```python
from build123d import *

# Parameters (mm, degrees)
SKETCH1_W           = 30
SKETCH1_H           = 239.95
BOSS_EXTRUDE1_DEPTH = 3.75
SKETCH2_W           = 30
SKETCH2_H           = 5
BOSS_EXTRUDE2_DEPTH = 20
SKETCH3_W           = 30
SKETCH3_H           = 5
BOSS_EXTRUDE3_DEPTH = 20
FILLET1_R           = 10
FILLET2_R           = 10


with BuildPart() as part:
    # Sketch1 → Boss-Extrude1 (new body, symmetric)
    with BuildSketch(Plane.XY):
        with Locations((0, 119.975)):
            Rectangle(SKETCH1_W, SKETCH1_H)
    extrude(amount=BOSS_EXTRUDE1_DEPTH, both=True)

    # Sketch2 → Boss-Extrude2 (add, symmetric)
    with BuildSketch(Plane.XY):
        with Locations((0, 2.5)):
            Rectangle(SKETCH2_W, SKETCH2_H)
    extrude(amount=BOSS_EXTRUDE2_DEPTH, both=True)

    # Sketch3 → Boss-Extrude3 (add, symmetric)
    with BuildSketch(Plane.XY):
        with Locations((0, 237.45)):
            Rectangle(SKETCH3_W, SKETCH3_H)
    extrude(amount=BOSS_EXTRUDE3_DEPTH, both=True)

    # Fillet1
    fillet1_edges = [part.edges().sort_by_distance(p)[0] for p in [
        (0, 234.95, 3.75),
        (0, 234.95, -3.75),
    ]]
    fillet(fillet1_edges, radius=FILLET1_R)

    # Fillet2
    fillet2_edges = [part.edges().sort_by_distance(p)[0] for p in [
        (0, 5, -3.75),
        (0, 5, 3.75),
    ]]
    fillet(fillet2_edges, radius=FILLET2_R)


solid = part.part
```
CAD build for the part. Positions are in the model's coordinates, mm. A direction names the side the tool comes from. Give positions to 0.01 mm unless a question says otherwise; leave off trailing zeros. Loops run counter-clockwise (first coordinate to the right, second up) from the corner with the lowest first, then second, coordinate; pieces in that order, holes last. Notation, with made-up numbers: (-27, 19.5) - (32, 19.5) arc R19 cw to (32, 31.5) - close; hole circle Ø9 at (27, 71). An arc over 180 degrees is marked (long way). Put each result on its own line as item: value.
Q1. Slice it at C-C (y = 46.5). Give the cut face in (x, z), plus the area to 3 significant figures.
Filled in:
outline: (-15, -3.75) - (15, -3.75) - (15, 3.75) - (-15, 3.75) - close
area: 225 mm²
Q2. Mould opens along X. For faces 4 (the face through (15, 111, 0)), 5 (the face through (0, 5, 17)), 6 (the face through (-15, 111, 0)) say: pulls with the +X half, pulls with the -X half, needs draft (parallel to the pull), parting line crosses it, or undercut.
Filled in:
face 4: pulls with the +X half
face 5: needs draft
face 6: pulls with the -X half
Q3. Probe line 1 along Y through (x, z) = (-8.25, 15); line 2 along Z through (x, y) = (8.25, 180); line 3 along Y through (x, z) = (-5.5, -11). List the from-to ranges inside material, lowest first.
Filled in:
line 1: y = 0 to 5, 234.95 to 239.95
line 2: z = -3.75 to 3.75
line 3: y = 0 to 5.39, 234.56 to 239.95
Q4. Slice it at B-B (z = -17). Give the cut face in (x, y).
Filled in:
outline: (-15, 0) - (15, 0) - (15, 5) - (-15, 5) - close; (-15, 234.95) - (15, 234.95) - (15, 239.95) - (-15, 239.95) - close
Q5. Tool access for faces 1 (the face through (0, 3, -20)), 2 (the face through (0, 234.95, 17)), 3 (the face through (0, 121, -3.75)): list every direction of +Z, -Z, +X, -X, +Y, -Y with a clear straight run to the whole face (end or side of a thin tool).
Filled in:
face 1: -Z, +X, -X, +Y, -Y
face 2: +Z, +X, -X
face 3: -Z, +X, -X
Q6. Flat gauge pins, fed straight in: pin 1 (8 mm diameter, centred on x = -9.5, y = 194.5, fed in from +Z); pin 2 (9 mm diameter, centred on x = -6.5, y = 127.5, fed in from -Z). Where does each tip first touch, or does it go through?
Filled in:
pin 1: stops at z = 3.75
pin 2: stops at z = -3.75
Q7. Slice it at A-A (x = -5.5). Give the cut face in (y, z).
Filled in:
outline: (0, -20) - (5, -20) - (5, -13.75) arc R10 cw to (15, -3.75) - (224.95, -3.75) arc R10 cw to (234.95, -13.75) - (234.95, -20) - (239.95, -20) - (239.95, 20) - (234.95, 20) - (234.95, 13.75) arc R10 cw to (224.95, 3.75) - (15, 3.75) arc R10 cw to (5, 13.75) - (5, 20) - (0, 20) - close
